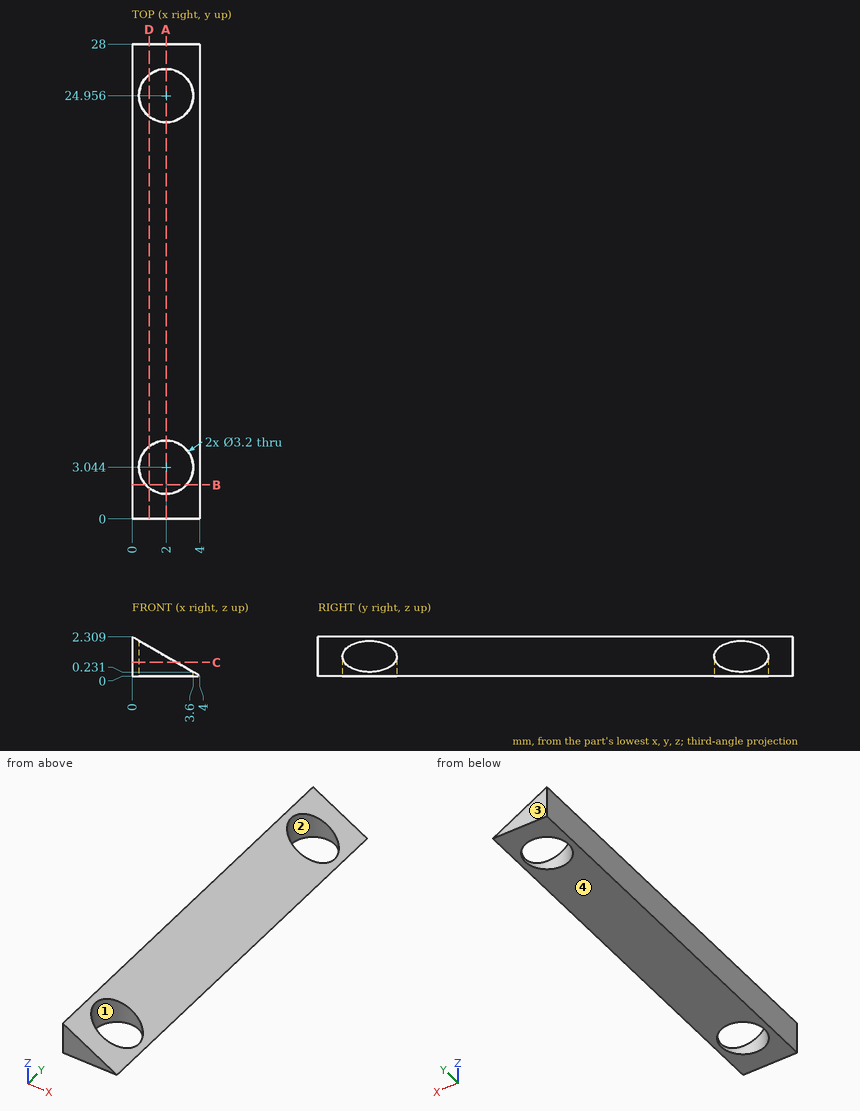
Check sheet for the drawn part. Datum: minimum x, y, z corner. Units: mm. Give positions to 0.01 mm unless a question says otherwise; leave off trailing zeros. Order: outer loops, then holes, each group sorted by start corner. A loop starts at its lowest first (then second) coordinate and runs counter-clockwise, first axis right, second up. Notation, with made-up numbers: (51.5, 29.5) - (96.5, 29.5) arc R25 cw to (96.5, 53.5) - close; hole circle Ø10 at (-19.75, -17.75). An arc over 180 degrees is marked (long way). Write item = value, one per line. Start each with the question number.
1) Section check B-B (y = 2). Enter the section's corners in (x, z) (1 decimal).
2) Draft check along Y on the marked faces 1, 2, 3 and 4. Enter one of: released by +Y, released by -Y, zero draft, split by the parting line, or undercut.
3) Section check A-A (x = 2). Enter the section's corners in (y, z) (1 decimal).
4) Scan lines: L1, parallel to Y at x = 2, z = 0.4; L2, parallel to Y at x = 2.6, z = 0.4; L3, parallel to Z at x = 0.4, y = 16.25. Record each from-to range of solid material in increasing order.
5) Section check C-C (z = 0.8). Enter the section's corners in (x, y) (1 decimal).
6) Section check D-D (x = 1). Enter the section's corners in (y, z) (1 decimal).
Geometry check:
q1.outline = (0, 0) - (0.8, 0) - (0.8, 1.9) - (0, 2.3) - close; (3.2, 0) - (4, 0) - (3.2, 0.5) - close
q2.face_1 = undercut
q2.face_2 = undercut
q2.face_3 = released by +Y
q2.face_4 = zero draft
q3.outline = (0, 0) - (1.4, 0) - (1.4, 1.2) - (0, 1.2) - close; (4.6, 0) - (23.4, 0) - (23.4, 1.2) - (4.6, 1.2) - close; (26.6, 0) - (28, 0) - (28, 1.2) - (26.6, 1.2) - close
q4.L1 = 0 to 1.44, 4.64 to 23.36, 26.56 to 28
q4.L2 = 0 to 1.56, 4.53 to 23.47, 26.44 to 28
q4.L3 = 0 to 2.08
q5.outline = (0, 0) - (2.6, 0) - (2.6, 1.6) arc R1.6 cw (long way) to (2.6, 4.5) - (2.6, 23.5) arc R1.6 cw (long way) to (2.6, 26.4) - (2.6, 28) - (0, 28) - close
q6.outline = (0, 0) - (1.8, 0) - (1.8, 1.7) - (0, 1.7) - close; (4.3, 0) - (23.7, 0) - (23.7, 1.7) - (4.3, 1.7) - close; (26.2, 0) - (28, 0) - (28, 1.7) - (26.2, 1.7) - close
